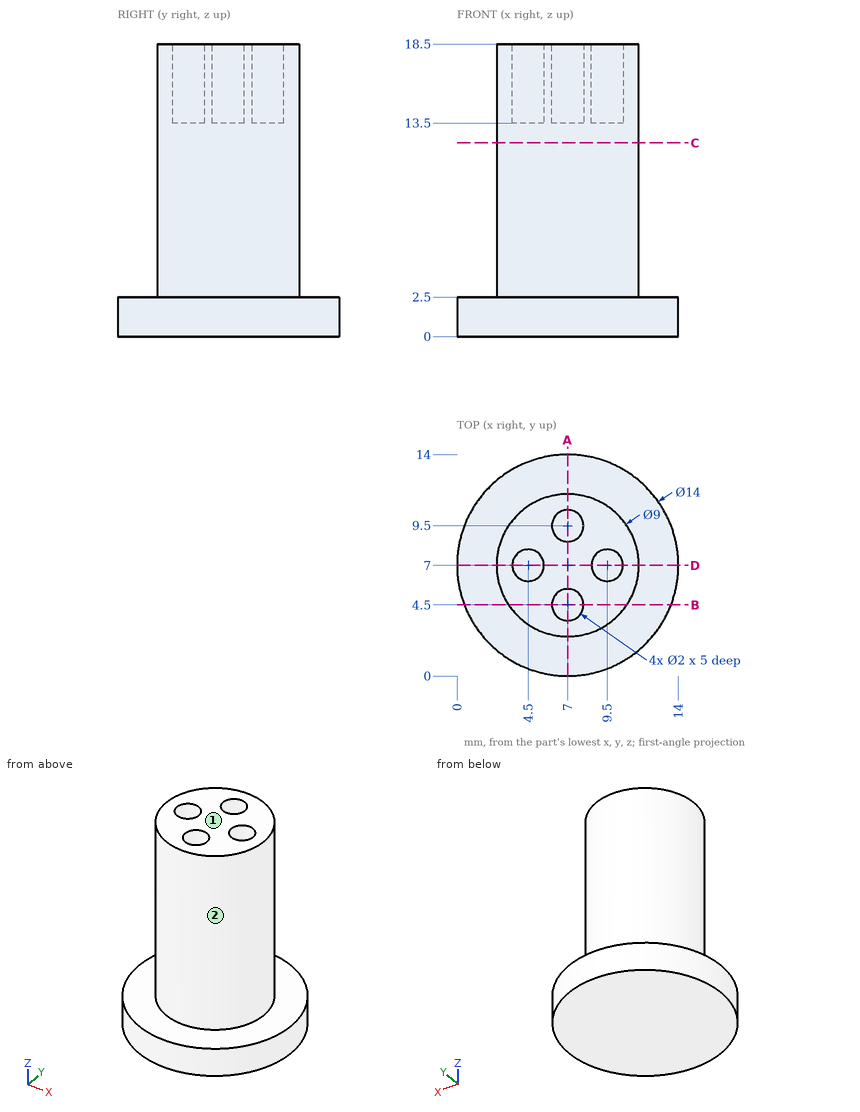
Could you check a few things on this drawing? It's one solid part, dimensions in mm from its lowest x, y, z. A direction names the side the tool comes from. Give positions to 0.01 mm unless a question says otherwise; leave off trailing zeros. Order: outer loops, then holes, each group sorted by start corner. A loop starts at its lowest first (then second) coordinate and runs counter-clockwise, first axis right, second up. Notation, with made-up numbers: (-29, -31.75) - (24, -31.75) arc R29 ccw to (24, -5.75) - close; hole circle Ø8 at (-17.5, 56). An arc over 180 degrees is marked (long way). One line per question, with ' | ' between items. Start each with the question number.
Item 1: I need wall thicknesses on probe 1 along Y at (x, z) = (7, 15.5); probe 2 along Z at (x, y) = (3.75, 10.75); probe 3 along X at (y, z) = (8.75, 16.25). Which ranges of each line are inside material? Lowest first, please. Write a range as [from, to].
Item 2: I'm going to push flat-ended pins straight in: pin 1 Ø8 at (x, z) = (12, 8) entering from -Y; pin 2 Ø1.8 at (x, y) = (9.5, 7) entering from +Z; pin 3 Ø1.2 at (x, y) = (4.5, 7) entering from -Z; pin 4 Ø5 at (x, z) = (4, 15) entering from +Y. Where does each tip first touch, or does it pass through?
Item 3: For the marked faces 1 and 2, which set-ups out of +Z, -Z, +X, -X, +Y, -Y let a thin tool reach every point of the face, with its end or its side?
Item 4: I want a section at C-C on z = 12.25. Write out the boundary of the cut face in (x, y), then the cut area to 3 significant figures.
Item 5: I want a section at B-B on y = 4.5. Write out the boundary of the cut face in (x, z).
Item 6: I want a section at A-A on x = 7. Write out the boundary of the cut face in (y, z), then the cut area to 3 significant figures.
Verdict:
1) probe 1: [2.5, 3.5], [5.5, 8.5], [10.5, 11.5] | probe 2: [0, 2.5] | probe 3: [2.85, 6.34], [7.66, 11.15]
2) pin 1: y = 2.61 | pin 2: z = 13.5 | pin 3: z = 0 | pin 4: y = 11.47
3) face 1: +Z, +X, -X, +Y, -Y | face 2: +Z
4) outline: circle Ø9 at (7, 7) | area: 63.6 mm^2
5) outline: (0.46, 0) - (13.54, 0) - (13.54, 2.5) - (10.74, 2.5) - (10.74, 18.5) - (8, 18.5) - (8, 13.5) - (6, 13.5) - (6, 18.5) - (3.26, 18.5) - (3.26, 2.5) - (0.46, 2.5) - close
6) outline: (0, 0) - (14, 0) - (14, 2.5) - (11.5, 2.5) - (11.5, 18.5) - (10.5, 18.5) - (10.5, 13.5) - (8.5, 13.5) - (8.5, 18.5) - (5.5, 18.5) - (5.5, 13.5) - (3.5, 13.5) - (3.5, 18.5) - (2.5, 18.5) - (2.5, 2.5) - (0, 2.5) - close | area: 159 mm^2
